The listing builds one solid part. Answer for the finished solid, in the listing's coordinates (mm). A direction names the side the tool comes from. Give positions to 0.01 mm unless a question says otherwise; leave off trailing zeros. Loops run counter-clockwise (first coordinate to the right, second up) from the corner with the lowest first, then second, coordinate; pieces in that order, holes last. Notation, with made-up numbers: M 31,85.5 L 54,85.5 A12 cw 54,94.5 Z; hole C 35,-38.75 d5. An arc over 180 degrees is marked long. Return JSON: item names as keys, results as strings.
from build123d import *

# Parameters (mm, degrees)
F0_W     = 50
F0_H     = 52
F0_W_2   = 1.5
F0_H_2   = 9.7
F1_DEPTH = 5
F2_R     = 5.9215
F3_DEPTH = 1.6
F4_R     = 3.0875
F5_DEPTH = 5.001


with BuildPart() as f1:
    # F0 (on Front) → F1 (new body)
    with BuildSketch(Plane.XZ):
        Rectangle(F0_W, F0_H)
        with Locations((-21.75, 4)):
            Rectangle(F0_W_2, F0_H_2, mode=Mode.SUBTRACT)
        with Locations((21.75, 4)):
            Rectangle(F0_W_2, F0_H_2, mode=Mode.SUBTRACT)
    extrude(amount=F1_DEPTH)

    # F2 (on Front) → F3 (cut)
    with BuildSketch(Plane.XZ):
        with Locations((7.5, 7.5)):
            Circle(F2_R)
        with Locations((7.5, -7.5)):
            Circle(F2_R)
        with Locations((-7.5, -7.5)):
            Circle(F2_R)
        with Locations((-7.5, 7.5)):
            Circle(F2_R)
    extrude(amount=F3_DEPTH, mode=Mode.SUBTRACT)

    # F4 (on Front) → F5 (cut, through all)
    with BuildSketch(Plane.XZ):
        with Locations((7.5, 7.5)):
            Circle(F4_R)
        with Locations((-7.5, 7.5)):
            Circle(F4_R)
        with Locations((-7.5, -7.5)):
            Circle(F4_R)
        with Locations((7.5, -7.5)):
            Circle(F4_R)
    extrude(amount=F5_DEPTH, mode=Mode.SUBTRACT)


solid = f1.part
(1) A tool of negligible diameter and unlimited length cuts with its end or side. For faces 1 (the flat face through (-22.5, -2, 4)), 2 (the flat face through (-5, -1.6, -10)), 3 (the flat face through (0, -2, -26)), from which of +Z, -Z, +X, -X, +Y, -Y can it reach the whole face along a straight path? Write none if from no direction.
Values follow:
{"face 1": "+Y, -Y", "face 2": "+Y", "face 3": "-Z, +X, -X, +Y, -Y"}
(2) The part is cut by section C-C (x = -7.5). Determine the outline of the cut face in (y, z).
Values follow:
{"outline": "M -5,-26 L 0,-26 L 0,-13.42 L -1.6,-13.42 L -1.6,-10.59 L -5,-10.59 Z; M -5,-4.41 L -1.6,-4.41 L -1.6,-1.58 L 0,-1.58 L 0,1.58 L -1.6,1.58 L -1.6,4.41 L -5,4.41 Z; M -5,10.59 L -1.6,10.59 L -1.6,13.42 L 0,13.42 L 0,26 L -5,26 Z"}
(3) The part is cut by section A-A (y = -3). Give the number of separate pieces and of enclosed holes in the cut face, and give its area (3 significant figures).
Values follow:
{"separate pieces": "1", "enclosed holes": "6", "area": "2,450 mm²"}
(4) Determine the mould class of faces 4 (the flat face through (-22, -2, 8.85)), 5 (the flat face through (25, -2, 0)), 6 (the flat face through (0, 0, 0)) for opening direction X: released by +X, released by -X, zero draft, split by the parting line, or undercut.
Values follow:
{"face 4": "undercut", "face 5": "released by +X", "face 6": "zero draft"}
(5) The part is cut by section D-D (z = 7.5). Determine the outline of the cut face in (x, y), and give its area (3 significant figures).
Values follow:
{"outline": "M -25,-5 L -22.5,-5 L -22.5,0 L -25,0 Z; M -21,-5 L -10.59,-5 L -10.59,-1.6 L -13.42,-1.6 L -13.42,0 L -21,0 Z; M -4.41,-5 L 4.41,-5 L 4.41,-1.6 L 1.58,-1.6 L 1.58,0 L -1.58,0 L -1.58,-1.6 L -4.41,-1.6 Z; M 10.59,-5 L 21,-5 L 21,0 L 13.42,0 L 13.42,-1.6 L 10.59,-1.6 Z; M 22.5,-5 L 25,-5 L 25,0 L 22.5,0 Z", "area": "155 mm²"}
(6) Straight lines are drawn through the part: line 1 along X through (y, z) = (-2.3, 0); line 2 along X through (y, z) = (-2.35, 7.5); line 3 along Z through (x, y) = (-7.5, -0.55). For each, find the intervals that lie inside material, in ascending order.
Values follow:
{"line 1": "-25 to -22.5, -21 to 21, 22.5 to 25", "line 2": "-25 to -22.5, -21 to -10.59, -4.41 to 4.41, 10.59 to 21, 22.5 to 25", "line 3": "-26 to -13.42, -1.58 to 1.58, 13.42 to 26"}
(7) The part is cut by section B-B (z = -7.5). Determine the outline of the cut face in (x, y), and give its area (3 significant figures).
Values follow:
{"outline": "M -25,-5 L -10.59,-5 L -10.59,-1.6 L -13.42,-1.6 L -13.42,0 L -25,0 Z; M -4.41,-5 L 4.41,-5 L 4.41,-1.6 L 1.58,-1.6 L 1.58,0 L -1.58,0 L -1.58,-1.6 L -4.41,-1.6 Z; M 10.59,-5 L 25,-5 L 25,0 L 13.42,0 L 13.42,-1.6 L 10.59,-1.6 Z", "area": "170 mm²"}
(8) Given pin 1 (3.5 mm diameter, centred on x = -7, z = -7, fed in from +Y); pin 2 (15.5 mm diameter, centred on x = -7.5, z = 7.5, fed in from +Y); pin 3 (10.5 mm diameter, centred on x = -7.5, z = -7.5, fed in from +Y), each flat-ended and moving along its own axis, determine where each tip first touches the part or whether it passes through.
Values follow:
{"pin 1": "through", "pin 2": "y = 0", "pin 3": "y = -1.6"}
